Autodesk Inventor part; units mm, degrees
ref_plane "YZ Plane" through (0, 0, 0) normal (1, 0, 0) x (0, 1, 0)
ref_plane "XZ Plane" through (0, 0, 0) normal (0, 1, 0) x (-1, 0, 0)
ref_plane "XY Plane" through (0, 0, 0) normal (0, 0, 1) x (1, 0, 0)
sketch "Эскиз1" plane through (0, 0, 0) normal (0, 1, 0) x (-1, 0, 0)
  line L0 (7.5, 22) -> (-7.5, 22)
  line L1 (-7.5, 22) -> (-7.5, -22)
  line L2 (-7.5, -22) -> (7.5, -22)
  line L3 (7.5, -22) -> (7.5, 22)
  line L4 (-7.5, 22) -> (7.5, -22) construction
  line L5 (0, 22) -> (0, -22) construction
  circle A0 centre (0, 16) radius 2
  line L6 (7.5, 0) -> (-7.5, 0) construction
  circle A1 centre (0, -16) radius 2
  point P0 (0, 0)
  point P1 (0, 0)
  dimension "d0" = 15
  dimension "d1" = 44
  dimension "d2" = 16
  dimension "d3" = 4
extrude "Выдавливание1" add sketch "Эскиз1" along normal blind 15.5
sketch "Эскиз2" plane through (7.5, 0, 22) normal (1, 0, 0) x (0, 0, -1)
  line L0 (0, 15.5) -> (44, 15.5)
  circle A0 centre (22, 15.5) radius 10.15
  point P0 (22, 0)
  dimension "Диаметр_мотора" = 20.3
extrude "Выдавливание2" cut sketch "Эскиз2" against normal through all
sketch "Эскиз4" plane through (0, 15.5, 0) normal (0, 1, 0) x (1, 0, 0)
  circle A0 centre (0, 16) radius 3.5
  circle A1 centre (0, 16) radius 2
  line L0 (-6, 12.5) -> (6, 12.5)
  line L1 (6, 16) -> (6, 0)
  line L2 (6, 0) -> (-6, 0)
  line L3 (-6, 0) -> (-6, 16)
  line L4 (-6, 12.5) -> (6, 0) construction
  line L5 (0, 0) -> (0, 16) construction
  arc A2 (6, 16) -> (-6, 16) centre (0, 16) ccw
  line L6 (7.5, 22) -> (-7.5, 22)
  line L7 (6, -16) -> (6, 0)
  line L8 (-6, 0) -> (-6, -16)
  arc A3 (-6, -16) -> (6, -16) centre (0, -16) ccw
  line L9 (7.5, 22) -> (-7.5, 22)
  line L10 (7.5, -22) -> (7.5, 22)
  line L11 (-7.5, 22) -> (7.5, 22)
  line L12 (7.5, 22) -> (7.5, -22)
  line L13 (7.5, -22) -> (-7.5, -22)
  line L14 (-7.5, -22) -> (-7.5, 22)
  point P0 (0, 6.25)
  point P1 (0, 12.5)
  point P2 (0, 22)
  point P3 (0, -22)
  dimension "d12" = 7
extrude "Выдавливание3" cut sketch "Эскиз4" against normal through all contours L3 L8 A3 L13 L14 L6 A2 | L1 A2 L6 L10 L13 A3 L7
properties part number "motor_mount_edge_part2"
Source: CAD feature listing. Evaluate the final solid. Frame: model axes, mm. Round coordinates to 2 decimals unless told otherwise and drop trailing zeros. Write each loop counter-clockwise with the first axis right and the second up, starting at its lowest first coordinate (ties: lowest second). Pieces come first, ordered by that corner, then holes. Notation, with made-up numbers: M 87.25,55 L 137.25,55 A24 ccw 137.25,87 Z; hole C 53,-34 d2. An arc over 180 degrees is marked long. Answer as a JSON object with one key per item and string values. Group by question number.
(1) First-contact query: pin 1 (4 mm diameter, centred on x = -2.5, z = 4.5, fed in from +Y); pin 2 (3 mm diameter, centred on x = 0, z = 16, fed in from -Y); pin 3 (5 mm diameter, centred on x = -4.5, y = 3.5, fed in from +Z). Flat tips, straight axial feed; report the tip coordinate or a pass-through.
(2) Ray query, line 1 (Z direction, x = 0, y = 7.25); line 2 (Z direction, x = 0, y = 9.25); line 3 (Z direction, x = 2.75, y = 7.75). Return the intervals inside material, ascending. Write a range as [from, to].
(3) Section query C-C on y = 1. Output: boundary loops of the cut face in (x, z), then the cut area to 3 significant figures.
(4) Mould query, pull axis Z, two halves, no side actions, for faces 1 (the flat face through (0.1, 15.5, 13.5)), 2 (the cylindrical face through (0, 8, 14)), 3 (the cylindrical face through (0, 8, 22)). Classes: +Z half, -Z half, draft (parallel to the pull), parting line (faces both ways), or undercut.
(5) Section query D-D on x = 2.75. Output: boundary loops of the cut face in (y, z).
(6) Section query B-B on y = 12.25. Output: boundary loops of the cut face in (x, z).
(7) Section query A-A on x = 0. Output: boundary loops of the cut face in (y, z).
Computed values:
{
 "1": {"pin 1": "y = 7.7", "pin 2": "through", "pin 3": "z = 21.66"},
 "2": {"line 1": "[-22, -18], [-14, -5.91], [5.91, 14], [18, 22]", "line 2": "[-22, -18], [-14, -8], [8, 14], [18, 22]", "line 3": "[-21.33, -6.55], [6.55, 21.33]"},
 "3": {"outline": "M -6,-16 A6 ccw 6,-16 L 6,16 A6 ccw -6,16 Z; hole C 0,-16 d4; hole C 0,16 d4", "area": "472 mm^2"},
 "4": {"face 1": "draft", "face 2": "undercut", "face 3": "+Z half"},
 "5": {"outline": "M 0,-21.33 L 15.5,-21.33 L 15.5,-10.15 A10.15 cw 15.5,10.15 L 15.5,21.33 L 0,21.33 Z"},
 "6": {"outline": "M -6,-16 A6 ccw 6,-16 L 6,-9.62 L -6,-9.62 Z; M -6,9.62 L 6,9.62 L 6,16 A6 ccw -6,16 Z; hole C 0,-16 d4; hole C 0,16 d4"},
 "7": {"outline": "M 0,-22 L 15.5,-22 L 15.5,-18 L 0,-18 Z; M 0,-14 L 15.5,-14 L 15.5,-10.15 A10.15 cw 15.5,10.15 L 15.5,14 L 0,14 Z; M 0,18 L 15.5,18 L 15.5,22 L 0,22 Z"}
}
